Design review of the part built by this model. Coordinates are the model's own, in mm. A direction names the side the tool comes from. Give positions to 0.01 mm unless a question says otherwise; leave off trailing zeros. Loops run counter-clockwise (first coordinate to the right, second up) from the corner with the lowest first, then second, coordinate; pieces in that order, holes last. Notation, with made-up numbers: M 60,23 L 94,23 A14 cw 94,34 Z; hole C 7.5,-30.5 d4. An arc over 180 degrees is marked long. Use a Markdown table: item, result. Add a question column.
(1) For faces 1 (the face through (5.781, 12.538, -3.948)), 2 (the face through (0.05, -12.1, 9.28)), 3 (the face through (-5.749, 12.538, -3.948)), 4 (the face through (6.89, 6, 11)), 5 (the face through (4.27, 5.83, 11.21)), list the 3-axis set-ups (+Z, -Z, +X, -X, +Y, -Y) from which the entire face can be reached by the end or side of a thin tool; tool diameter is ignored.
(2) Insertion check: pin 1 Ø4 at (x, y) = (-3, 1) entering from +Z; pin 2 Ø1 at (x, z) = (-3, 10) entering from +Y. Each pin has a flat end and moves straight along its axis. Give the tip position at first contact, or say it passes through.
(3) Add section A-A, the plane z = 0. Give the boundary of the cut face in (x, y), then the cut area to 3 significant figures.
(4) For probe 1 along X at (y, z) = (10.5, 7.5); probe 2 along Z at (x, y) = (3, 0); probe 3 along Z at (x, y) = (3.5, -1.5), list the stretches that pass through material, from the lowest coordinate up.
(5) Add section C-C, the plane x = 2.5. Give the boundary of the cut face in (y, z).
(6) Draft analysis for pull direction Y (two halves, no side actions). For faces 6 (the face through (-4.64, -6.9, -10.8)), 7 (the face through (-0.096, -11.446, 3.604)), 8 (the face through (-4.26, 5.83, 11.21)), state which applies: pulls with the +Y half, pulls with the -Y half, needs draft (parallel to the pull), parting line crosses it, or undercut.
```python
from build123d import *

# Parameters (mm, degrees)
SKETCH3_R          = 12
CUT_EXTRUDE1_DEPTH = 26.593229573


with BuildPart() as part:
    # Sketch2 → Revolve1 (revolve)
    with BuildSketch(Plane.XY):
        Polygon((6.89, 0), (-6.89, 0), (-6.89, 13.1445), (-4.64, 13.1445), (-4.64, 12.6365), (-3.89, 12.6365), (-3.89, 15.25), (3.89, 15.25), (3.89, 12.6365), (4.64, 12.6365), (4.64, 13.1445), (6.89, 13.1445), align=None)
    revolve(axis=Axis((6.89, 0, 0), (-1, 0, 0)))

    # Sketch3 → Cut-Extrude1 (cut, through all)
    with BuildSketch(Plane.ZY.offset(6.89)):
        with Locations(Location((0, 0, 0), (0, 0, 270))):
            Circle(SKETCH3_R)
    extrude(amount=-CUT_EXTRUDE1_DEPTH, mode=Mode.SUBTRACT)


solid = part.part
```
Established:
| question | item | result |
|---|---|---|
| 1 | face 1 | +X |
| 1 | face 2 | +X, -X |
| 1 | face 3 | -X |
| 1 | face 4 | +Z, -Z, +X, +Y, -Y |
| 1 | face 5 | none |
| 2 | pin 1 | z = 15.25 |
| 2 | pin 2 | y = 11.93 |
| 3 | outline | M -6.89,-13.14 L -4.64,-13.14 L -4.64,-12.64 L -3.89,-12.64 L -3.89,-15.25 L 3.89,-15.25 L 3.89,-12.64 L 4.64,-12.64 L 4.64,-13.14 L 6.89,-13.14 L 6.89,-12 L -6.89,-12 Z; M -6.89,12 L 6.89,12 L 6.89,13.14 L 4.64,13.14 L 4.64,12.64 L 3.89,12.64 L 3.89,15.25 L -3.89,15.25 L -3.89,12.64 L -4.64,12.64 L -4.64,13.14 L -6.89,13.14 Z |
| 3 | area | 62.8 mm^2 |
| 4 | probe 1 | -6.89 to -4.64, -3.89 to 3.89, 4.64 to 6.89 |
| 4 | probe 2 | -15.25 to -12, 12 to 15.25 |
| 4 | probe 3 | -15.18 to -11.91, 11.91 to 15.18 |
| 5 | outline | C 0,0 d30.5; hole C 0,0 d24 |
| 6 | face 6 | needs draft |
| 6 | face 7 | undercut |
| 6 | face 8 | parting line crosses it |
